from build123d import *

# Parameters (mm, degrees)
F1_DEPTH = 5.08
F2_W     = 6.35
F2_H     = 33.02
F3_DEPTH = 5.08
F4_DEPTH = 12.7
F5_R     = 1.143
F6_DEPTH = 25.4
F7_W     = 45.72
F7_H     = 45.72
F7_W_2   = 33.02
F7_H_2   = 33.02
F8_DEPTH = 17.78


with BuildPart() as f1:
    # F0 (on Top) → F1 (new body)
    with BuildSketch(Plane.XY):
        Polygon((15.6999393499, 19.6573674963), (-17.3200606501, 19.6573674963), (-17.3200606501, -13.3626325037), (-4.6200606501, -13.3626325037), (-4.6200606501, -8.2826325037), (2.9999393499, -8.2826325037), (2.9999393499, -13.3626325037), (15.6999393499, -13.3626325037), align=None)
    extrude(amount=F1_DEPTH)

    # F2 (on face) → F3 (join)
    with BuildSketch(Plane.XY.offset(5.08)):
        with Locations((18.8749393499, 3.1473674963)):
            Rectangle(F2_W, F2_H)
        Polygon((-17.3200606501, 26.0073674963), (-17.3200606501, 19.6573674963), (15.6999393499, 19.6573674963), (22.0499393499, 19.6573674963), (22.0499393499, 26.0073674963), align=None)
        Polygon((-4.6200606501, -13.3626325037), (-17.3200606501, -13.3626325037), (-17.3200606501, -19.7126325037), (22.0499393499, -19.7126325037), (22.0499393499, -13.3626325037), (15.6999393499, -13.3626325037), (2.9999393499, -13.3626325037), align=None)
        Polygon((-17.3200606501, -13.3626325037), (-17.3200606501, 19.6573674963), (-17.3200606501, 26.0073674963), (-23.6700606501, 26.0073674963), (-23.6700606501, -19.7126325037), (-17.3200606501, -19.7126325037), align=None)
    extrude(amount=-F3_DEPTH)

    # F2 (on face) → F4 (join)
    with BuildSketch(Plane.XY.offset(5.08)):
        Polygon((-17.3200606501, 26.0073674963), (-17.3200606501, 19.6573674963), (15.6999393499, 19.6573674963), (22.0499393499, 19.6573674963), (22.0499393499, 26.0073674963), align=None)
        with Locations((18.8749393499, 3.1473674963)):
            Rectangle(F2_W, F2_H)
        Polygon((-4.6200606501, -13.3626325037), (-17.3200606501, -13.3626325037), (-17.3200606501, -19.7126325037), (22.0499393499, -19.7126325037), (22.0499393499, -13.3626325037), (15.6999393499, -13.3626325037), (2.9999393499, -13.3626325037), align=None)
        Polygon((-17.3200606501, -13.3626325037), (-17.3200606501, 19.6573674963), (-17.3200606501, 26.0073674963), (-23.6700606501, 26.0073674963), (-23.6700606501, -19.7126325037), (-17.3200606501, -19.7126325037), align=None)
    extrude(amount=F4_DEPTH)

    # F5 (on face) → F6 (cut)
    with BuildSketch(Plane.XY.offset(5.08)):
        with Locations((13.2869393499, 17.2443674963)):
            Circle(F5_R)
        with Locations((-14.9070606501, -10.9496325037)):
            Circle(F5_R)
        with Locations((13.2869393499, -10.9496325037)):
            Circle(F5_R)
        with Locations((-14.9070606501, 17.2443674963)):
            Circle(F5_R)
    extrude(amount=-F6_DEPTH, mode=Mode.SUBTRACT)

    # F7 (on face) → F8 (join)
    with BuildSketch(Plane.XY.offset(17.78)):
        with BuildLine():
            ThreePointArc((22.0499393499, -19.7126325037), (29.057968727, -9.224375353), (31.5188613857, 3.1473674963))
            ThreePointArc((31.5188613857, 3.1473674963), (29.057968727, 15.5191103457), (22.0499393499, 26.0073674963))
            Line((22.0499393499, 26.0073674963), (22.0499393499, -19.7126325037))
        make_face()
        with BuildLine():
            Line((-23.6700606501, 26.0073674963), (22.0499393499, 26.0073674963))
            ThreePointArc((22.0499393499, 26.0073674963), (-0.8100606501, 35.4762895322), (-23.6700606501, 26.0073674963))
        make_face()
        with Locations((-0.8100606501, 3.1473674963)):
            Rectangle(F7_W, F7_H)
        with Locations((-0.8100606501, 3.1473674963)):
            Rectangle(F7_W_2, F7_H_2, mode=Mode.SUBTRACT)
        with BuildLine():
            ThreePointArc((-23.6700606501, -19.7126325037), (-0.8100606501, -29.1815545395), (22.0499393499, -19.7126325037))
            Line((22.0499393499, -19.7126325037), (-23.6700606501, -19.7126325037))
        make_face()
        with BuildLine():
            Line((-23.6700606501, -19.7126325037), (-23.6700606501, 26.0073674963))
            ThreePointArc((-23.6700606501, 26.0073674963), (-33.138982686, 3.1473674963), (-23.6700606501, -19.7126325037))
        make_face()
    extrude(amount=-F8_DEPTH)


solid = f1.part
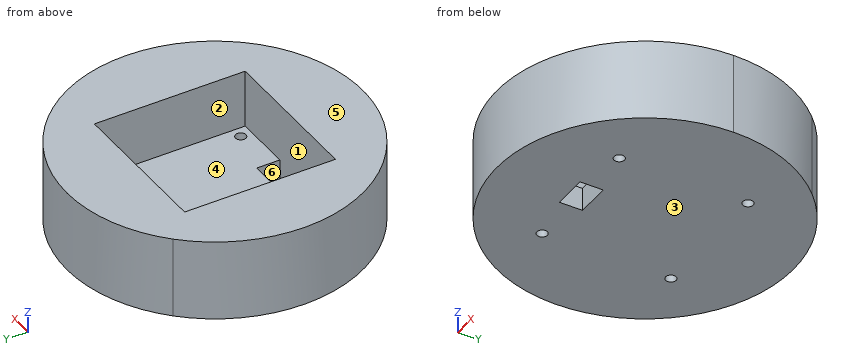
Source: CAD feature listing. Evaluate the final solid. Frame: model axes, mm. Face numbers are marked on the shaded views. A direction names the side the tool comes from. Coordinates: 2 decimals unless noted, no trailing zeros. Loops run counter-clockwise (first coordinate to the right, second up) from the corner with the lowest first, then second, coordinate; pieces in that order, holes last. Notation, with made-up numbers: (7, -13) - (41, -13) arc R21 cw to (41, 13) - close; hole circle Ø8 at (49.5, 75). An arc over 180 degrees is marked (long way). Return JSON: item names as keys, results as strings.
Q1. Contact query for flat-ended pins moving along their axis: P1, Ø4, axis at y = -11.5, z = 2, coming from the +X side; P2, Ø1.5, axis at y = 7, z = 5, coming from the -X side; P3, Ø1.5, axis at y = 17.5, z = 5, coming from the -X side. Output: stop coordinate, or through.
Results:
{"P1": "x = 28.94", "P2": "x = -32.99", "P3": "x = -30.14"}
Q2. Mould query, pull axis X, two halves, no side actions, for the marked faces 1, 2 and 3. Classes: released by +X, released by -X, zero draft, split by the parting line, or undercut.
Results:
{"face 1": "undercut", "face 2": "undercut", "face 3": "zero draft"}
Q3. Section B-B, the plane x = 13.5. Return loops of the section in (y, z), plus the area to 3 significant figures.
Results:
{"outline": "(-25.84, 0) - (-12.07, 0) - (-12.07, 5.08) - (-13.36, 5.08) - (-13.36, 17.78) - (-25.84, 17.78) - close; (-9.83, 0) - (16.12, 0) - (16.12, 5.08) - (-9.83, 5.08) - close; (18.37, 0) - (32.14, 0) - (32.14, 17.78) - (19.66, 17.78) - (19.66, 5.08) - (18.37, 5.08) - close", "area": "589 mm2"}
Q4. Section C-C, the plane x = 0. Return loops of the section in (y, z).
Results:
{"outline": "(-29.17, 0) - (-13.36, 0) - (-13.36, 17.78) - (-29.17, 17.78) - close; (-8.28, 0) - (35.47, 0) - (35.47, 17.78) - (19.66, 17.78) - (19.66, 5.08) - (-8.28, 5.08) - close"}
Q5. Material intervals for line 1 along Y through (x, z) = (0, 3); line 2 along Y through (x, z) = (-14, 2); line 3 along Z through (x, y) = (5, -0.5), sorted ascending.
Results:
{"line 1": "-29.17 to -13.36, -8.28 to 35.47", "line 2": "-26.37 to -11.65, -10.25 to 16.55, 17.94 to 32.66", "line 3": "0 to 5.08"}
Q6. Section A-A, the plane z = 6.25. Return loops of the section in (x, y), plus the area to 3 significant figures.
Results:
{"outline": "circle Ø64.66 at (-0.81, 3.15); hole (-17.32, -13.36) - (15.7, -13.36) - (15.7, 19.66) - (-17.32, 19.66) - close", "area": "2,190 mm2"}
Q7. Section D-D, the plane y = 6. Return loops of the section in (x, z).
Results:
{"outline": "(-33.01, 0) - (31.39, 0) - (31.39, 17.78) - (15.7, 17.78) - (15.7, 5.08) - (-17.32, 5.08) - (-17.32, 17.78) - (-33.01, 17.78) - close"}
Q8. Access query for the marked faces 4, 5 and 6. Directions: +Z, -Z, +X, -X, +Y, -Y. A direction counts if a zero-diameter tool reaches every point of the face in a straight line with its end or side. Return the directions, or none.
Results:
{"face 4": "+Z", "face 5": "+Z, +X, -X, +Y, -Y", "face 6": "+Z, -Z"}
